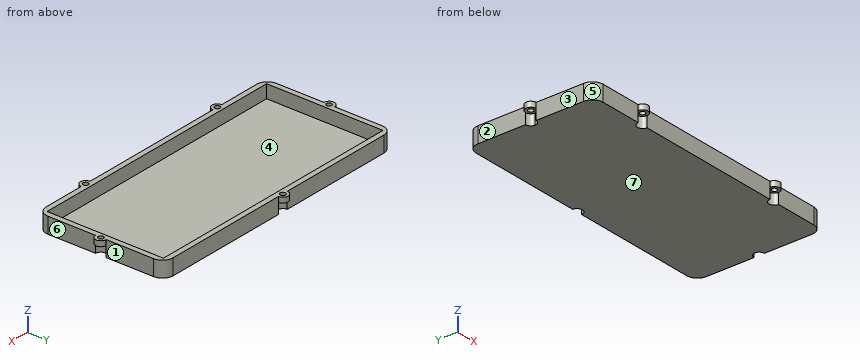
from build123d import *

# Parameters (mm, degrees)
CYLINDER022_R     = 2
CYLINDER022_DEPTH = 6
CYLINDER024_R     = 2
CYLINDER024_DEPTH = 6
CYLINDER023_R     = 2
CYLINDER023_DEPTH = 6
CYLINDER020_R     = 2
CYLINDER020_DEPTH = 6
CYLINDER021_R     = 2
CYLINDER021_DEPTH = 6
CYLINDER014_R     = 1
CYLINDER014_DEPTH = 13
CYLINDER012_R     = 1
CYLINDER012_DEPTH = 13
CYLINDER013_R     = 1
CYLINDER013_DEPTH = 13
CYLINDER011_R     = 1
CYLINDER011_DEPTH = 13
CYLINDER010_R     = 1
CYLINDER010_DEPTH = 13
BOX012_W          = 10
BOX012_H          = 17
BOX012_DEPTH      = 8
BOX010_W          = 10
BOX010_H          = 17
BOX010_DEPTH      = 8
BOX013_W          = 10
BOX013_H          = 17
BOX013_DEPTH      = 8
BOX009_W          = 10
BOX009_H          = 17
BOX009_DEPTH      = 8
BOX008_W          = 10
BOX008_H          = 17
BOX008_DEPTH      = 8
BOX011_W          = 100
BOX011_H          = 44
BOX011_DEPTH      = 16.5
BOX007_W          = 104
BOX007_H          = 48
BOX007_DEPTH      = 6
FILLET001_R       = 4
CYLINDER019_R     = 2
CYLINDER019_DEPTH = 6
CYLINDER018_R     = 2
CYLINDER018_DEPTH = 6
CYLINDER017_R     = 2
CYLINDER017_DEPTH = 6
CYLINDER016_R     = 2
CYLINDER016_DEPTH = 6
CYLINDER015_R     = 2
CYLINDER015_DEPTH = 6


with BuildPart() as cylinder022:
    # Cylinder022 → Cylinder022 (new body)
    with BuildSketch(Plane(origin=(-2, 22, 0), x_dir=(1, 0, 0), z_dir=(0, 0, 1))):
        Circle(CYLINDER022_R)
    extrude(amount=CYLINDER022_DEPTH)


with BuildPart() as cylinder024:
    # Cylinder024 → Cylinder024 (new body)
    with BuildSketch(Plane(origin=(48, 46, 0), x_dir=(1, 0, 0), z_dir=(0, 0, 1))):
        Circle(CYLINDER024_R)
    extrude(amount=CYLINDER024_DEPTH)


with BuildPart() as cylinder023:
    # Cylinder023 → Cylinder023 (new body)
    with BuildSketch(Plane(origin=(102, 22, 0), x_dir=(1, 0, 0), z_dir=(0, 0, 1))):
        Circle(CYLINDER023_R)
    extrude(amount=CYLINDER023_DEPTH)


with BuildPart() as cylinder020:
    # Cylinder020 → Cylinder020 (new body)
    with BuildSketch(Plane(origin=(80, -2, 0), x_dir=(1, 0, 0), z_dir=(0, 0, 1))):
        Circle(CYLINDER020_R)
    extrude(amount=CYLINDER020_DEPTH)


with BuildPart() as fusion005:
    # Cylinder021 → Cylinder021 (new body)
    with BuildSketch(Plane(origin=(20, -2, 0), x_dir=(1, 0, 0), z_dir=(0, 0, 1))):
        Circle(CYLINDER021_R)
    extrude(amount=CYLINDER021_DEPTH)

    # Fusion005: union Cylinder022, Cylinder024, Cylinder023, Cylinder020
    add(cylinder022.part)
    add(cylinder024.part)
    add(cylinder023.part)
    add(cylinder020.part)


with BuildPart() as fusion005_1:
    # Fusion005 placement: moved
    add(fusion005.part.moved(Location((0, 0, -8))))


with BuildPart() as cylinder014:
    # Cylinder014 → Cylinder014 (new body)
    with BuildSketch(Plane(origin=(-2, 22, 0), x_dir=(1, 0, 0), z_dir=(0, 0, 1))):
        Circle(CYLINDER014_R)
    extrude(amount=CYLINDER014_DEPTH)


with BuildPart() as cylinder012:
    # Cylinder012 → Cylinder012 (new body)
    with BuildSketch(Plane(origin=(48, 46, 0), x_dir=(1, 0, 0), z_dir=(0, 0, 1))):
        Circle(CYLINDER012_R)
    extrude(amount=CYLINDER012_DEPTH)


with BuildPart() as cylinder013:
    # Cylinder013 → Cylinder013 (new body)
    with BuildSketch(Plane(origin=(102, 22, 0), x_dir=(1, 0, 0), z_dir=(0, 0, 1))):
        Circle(CYLINDER013_R)
    extrude(amount=CYLINDER013_DEPTH)


with BuildPart() as cylinder011:
    # Cylinder011 → Cylinder011 (new body)
    with BuildSketch(Plane(origin=(80, -2, 0), x_dir=(1, 0, 0), z_dir=(0, 0, 1))):
        Circle(CYLINDER011_R)
    extrude(amount=CYLINDER011_DEPTH)


with BuildPart() as fusion003:
    # Cylinder010 → Cylinder010 (new body)
    with BuildSketch(Plane(origin=(20, -2, 0), x_dir=(1, 0, 0), z_dir=(0, 0, 1))):
        Circle(CYLINDER010_R)
    extrude(amount=CYLINDER010_DEPTH)

    # Fusion003: union Cylinder014, Cylinder012, Cylinder013, Cylinder011
    add(cylinder014.part)
    add(cylinder012.part)
    add(cylinder013.part)
    add(cylinder011.part)


with BuildPart() as fusion003_1:
    # Fusion003 placement: moved
    add(fusion003.part.moved(Location((0, 0, -6))))


with BuildPart() as box012:
    # Box012 → Box012 (new body)
    with BuildSketch(Plane(origin=(1.6, 37, 0), x_dir=(1, 0, 0), z_dir=(0, 0, 1))):
        with Locations((5, 8.5)):
            Rectangle(BOX012_W, BOX012_H)
    extrude(amount=BOX012_DEPTH)


with BuildPart() as box010:
    # Box010 → Box010 (new body)
    with BuildSketch(Plane(origin=(13.8, 37, 0), x_dir=(1, 0, 0), z_dir=(0, 0, 1))):
        with Locations((5, 8.5)):
            Rectangle(BOX010_W, BOX010_H)
    extrude(amount=BOX010_DEPTH)


with BuildPart() as box013:
    # Box013 → Box013 (new body)
    with BuildSketch(Plane(origin=(25.8, 37, 0), x_dir=(1, 0, 0), z_dir=(0, 0, 1))):
        with Locations((5, 8.5)):
            Rectangle(BOX013_W, BOX013_H)
    extrude(amount=BOX013_DEPTH)


with BuildPart() as box009:
    # Box009 → Box009 (new body)
    with BuildSketch(Plane(origin=(58.8, 37, 0), x_dir=(1, 0, 0), z_dir=(0, 0, 1))):
        with Locations((5, 8.5)):
            Rectangle(BOX009_W, BOX009_H)
    extrude(amount=BOX009_DEPTH)


with BuildPart() as box008:
    # Box008 → Box008 (new body)
    with BuildSketch(Plane(origin=(93.8, 42, 0), x_dir=(0, -1, 0), z_dir=(0, 0, 1))):
        with Locations((5, 8.5)):
            Rectangle(BOX008_W, BOX008_H)
    extrude(amount=BOX008_DEPTH)


with BuildPart() as fusion001:
    # Box011 → Box011 (new body)
    with BuildSketch(Plane.XY.offset(-5)):
        with Locations((50, 22)):
            Rectangle(BOX011_W, BOX011_H)
    extrude(amount=BOX011_DEPTH)

    # Fusion001: union Box012, Box010, Box013, Box009, Box008
    add(box012.part)
    add(box010.part)
    add(box013.part)
    add(box009.part)
    add(box008.part)


with BuildPart() as fillet001:
    # Box007 → Box007 (new body)
    with BuildSketch(Plane(origin=(-2, -2, -6), x_dir=(1, 0, 0), z_dir=(0, 0, 1))):
        with Locations((52, 24)):
            Rectangle(BOX007_W, BOX007_H)
    extrude(amount=BOX007_DEPTH)

    # Cut001: cut Fusion001
    add(fusion001.part, mode=Mode.SUBTRACT)

    # Fillet001
    fillet001_edges = [fillet001.edges().sort_by_distance(p)[0] for p in [
        (-2, -2, -3),
        (-2, 46, -3),
        (102, -2, -3),
        (102, 46, -3),
    ]]
    fillet(fillet001_edges, radius=FILLET001_R)


with BuildPart() as cylinder019:
    # Cylinder019 → Cylinder019 (new body)
    with BuildSketch(Plane(origin=(-2, 22, 0), x_dir=(1, 0, 0), z_dir=(0, 0, 1))):
        Circle(CYLINDER019_R)
    extrude(amount=CYLINDER019_DEPTH)


with BuildPart() as cylinder018:
    # Cylinder018 → Cylinder018 (new body)
    with BuildSketch(Plane(origin=(48, 46, 0), x_dir=(1, 0, 0), z_dir=(0, 0, 1))):
        Circle(CYLINDER018_R)
    extrude(amount=CYLINDER018_DEPTH)


with BuildPart() as cylinder017:
    # Cylinder017 → Cylinder017 (new body)
    with BuildSketch(Plane(origin=(102, 22, 0), x_dir=(1, 0, 0), z_dir=(0, 0, 1))):
        Circle(CYLINDER017_R)
    extrude(amount=CYLINDER017_DEPTH)


with BuildPart() as cylinder016:
    # Cylinder016 → Cylinder016 (new body)
    with BuildSketch(Plane(origin=(80, -2, 0), x_dir=(1, 0, 0), z_dir=(0, 0, 1))):
        Circle(CYLINDER016_R)
    extrude(amount=CYLINDER016_DEPTH)


with BuildPart() as cut008:
    # Cylinder015 → Cylinder015 (new body)
    with BuildSketch(Plane(origin=(20, -2, 0), x_dir=(1, 0, 0), z_dir=(0, 0, 1))):
        Circle(CYLINDER015_R)
    extrude(amount=CYLINDER015_DEPTH)

    # Fusion004: union Cylinder019, Cylinder018, Cylinder017, Cylinder016
    add(cylinder019.part)
    add(cylinder018.part)
    add(cylinder017.part)
    add(cylinder016.part)


with BuildPart() as cut008_1:
    # Fusion004 placement: moved
    add(cut008.part.moved(Location((0, 0, -6))))

    # Fusion006: union Fillet001
    add(fillet001.part)

    # Cut007: cut Fusion003
    add(fusion003_1.part, mode=Mode.SUBTRACT)

    # Cut008: cut Fusion005
    add(fusion005_1.part, mode=Mode.SUBTRACT)


solid = cut008_1.part
Model file for the job. Use its own axes, mm. Face numbers are marked on the shaded views. A direction names the side the tool comes from. Coordinates: 2 decimals unless noted, no trailing zeros. Order: outer loops, then holes, each group sorted by start corner. A loop starts at its lowest first (then second) coordinate and runs counter-clockwise, first axis right, second up. Notation, with made-up numbers: (-2.75, 27) -> (49.25, 27) arc R4 cw to (49.25, 33) -> close; hole circle Ø4 at (-7, 53). An arc over 180 degrees is marked (long way). Return JSON: item names as keys, results as strings. Group by question number.
Item 1: Wall check: line 1 along Y through (x, z) = (48, -0.6); line 2 along Y through (x, z) = (80, -1.35); line 3 along X through (y, z) = (22, -1.5). Give the ranges that are in metal, low to high. Write a range as [from, to].
Item 2: Saw through at B-B on y = 16. Write the cut outline in (x, z), then the cut area to 3 significant figures.
Item 3: Tool access for the marked faces 1, 2 and 3: list every direction of +Z, -Z, +X, -X, +Y, -Y with a clear straight run to the whole face (end or side of a thin tool).
Item 4: Saw through at C-C on x = 96. Write the cut outline in (y, z), then the cut area to 3 significant figures.
Item 5: Pull direction X, two halves, no side cores. Call the marked faces 4, 5, 6 and 7: pulls with the +X half, pulls with the -X half, needs draft (parallel to the pull), parting line crosses it, or undercut.
Item 6: Flat gauge pins, fed straight in: P1, Ø2, axis at x = 101.5, y = 21.5, coming from the -Z side; P2, Ø2.5, axis at x = 72, z = -2.5, coming from the +Y side; P3, Ø1, axis at y = 39.5, z = -4, coming from the +X side. Where does each tip first touch, or does it go through?
Values found:
{
 "1": {"line 1": "y = [-2, 0], [44, 45], [47, 48]", "line 2": "y = [-4, -3], [-1, 0], [44, 46]", "line 3": "x = [-4, -3], [-1, 0], [100, 101], [103, 104]"},
 "2": {"outline": "(-2, -6) -> (102, -6) -> (102, 0) -> (100, 0) -> (100, -5) -> (0, -5) -> (0, 0) -> (-2, 0) -> close", "area": "124 mm2"},
 "3": {"face 1": "+Z, -Z, +X, +Y", "face 2": "+Z, -Z, -X, +Y", "face 3": "+Z, -Z, -X, -Y"},
 "4": {"outline": "(-2, -6) -> (46, -6) -> (46, 0) -> (44, 0) -> (44, -5) -> (0, -5) -> (0, 0) -> (-2, 0) -> close", "area": "68.0 mm2"},
 "5": {"face 4": "undercut", "face 5": "pulls with the -X half", "face 6": "pulls with the +X half", "face 7": "needs draft"},
 "6": {"P1": "stops at z = -2", "P2": "stops at y = 46", "P3": "stops at x = 102"}
}
